Could you check a few things on this model? Use its own coordinates, in mm. Face numbers are marked on the shaded views. A direction names the side the tool comes from. Give positions to 0.01 mm unless a question says otherwise; leave off trailing zeros. Order: outer loops, then holes, each group sorted by start corner. A loop starts at its lowest first (then second) coordinate and runs counter-clockwise, first axis right, second up. Notation, with made-up numbers: (-14.5, 64) -> (-2.5, 64) arc R11 cw to (-2.5, 68) -> close; hole circle Ø6 at (47, 81). An arc over 180 degrees is marked (long way). One line per item, written item: value.
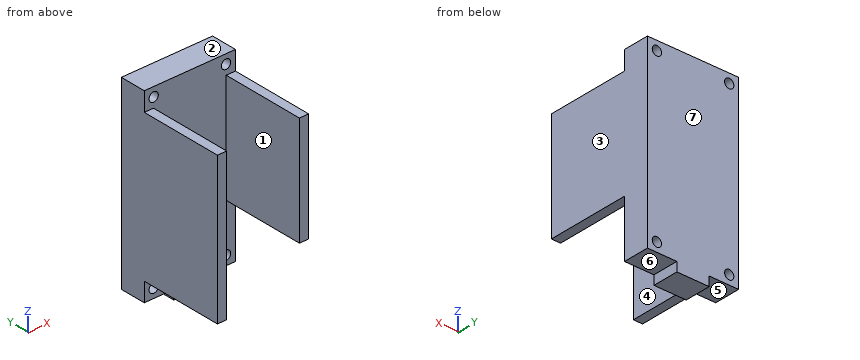
```python
from build123d import *

# Parameters (mm, degrees)
SKETCH1_W           = 25.0698
SKETCH1_H           = 51.054
SKETCH1_R           = 1.27
BOSS_EXTRUDE1_DEPTH = 7.1628
SKETCH2_W           = 2.54
SKETCH2_H           = 40.64
SKETCH2_H_2         = 30.1244
BOSS_EXTRUDE2_DEPTH = 22.86
SKETCH3_W           = 8.9
SKETCH3_H           = 7.1628
BOSS_EXTRUDE3_DEPTH = 2.54


with BuildPart() as part:
    # Sketch1 → Boss-Extrude1 (new body)
    with BuildSketch(Plane(origin=(0, 0, 0), x_dir=(1, 0, 0), z_dir=(0, 1, 0))):
        Rectangle(SKETCH1_W, SKETCH1_H)
        with Locations(Location((9.9441, 23.0124, 0), (0, 0, 270))):
            Circle(SKETCH1_R, mode=Mode.SUBTRACT)
        with Locations(Location((-9.9441, 23.0124, 0), (0, 0, 90))):
            Circle(SKETCH1_R, mode=Mode.SUBTRACT)
        with Locations(Location((9.9441, -23.0124, 0), (0, 0, 90))):
            Circle(SKETCH1_R, mode=Mode.SUBTRACT)
        with Locations(Location((-9.9441, -23.0124, 0), (0, 0, 270))):
            Circle(SKETCH1_R, mode=Mode.SUBTRACT)
    extrude(amount=BOSS_EXTRUDE1_DEPTH)

    # Sketch2 → Boss-Extrude2 (add)
    with BuildSketch(Plane.XZ):
        with Locations((-11.2649, 0)):
            Rectangle(SKETCH2_W, SKETCH2_H)
        with Locations((11.2649, 5.2578)):
            Rectangle(SKETCH2_W, SKETCH2_H_2)
    extrude(amount=BOSS_EXTRUDE2_DEPTH)

    # Sketch3 → Boss-Extrude3 (add)
    with BuildSketch(Plane(origin=(0, 0, -25.527), x_dir=(-1, 0, 0), z_dir=(0, 0, -1))):
        with Locations((0, 3.5814)):
            Rectangle(SKETCH3_W, SKETCH3_H)
    extrude(amount=BOSS_EXTRUDE3_DEPTH)


solid = part.part
```
1) If I drill on line 1 along X through (y, z) = (-6.5, 3.5); line 2 along Z through (x, y) = (-11, 5); line 3 along X through (y, z) = (-10.5, -16), over which ranges is the centre line in solid material (lowest first)?
Answer below:
line 1: x = -12.53 to -9.99, 9.99 to 12.53
line 2: z = -25.53 to -23.72, -22.31 to 22.31, 23.72 to 25.53
line 3: x = -12.53 to -9.99
2) We'd pull the mould along X, two halves only. Please class the marked faces 1, 2 and 3: +X half, -X half, draft (parallel to the pull), parting line (faces both ways), or undercut.
Answer below:
face 1: undercut
face 2: draft
face 3: +X half
3) Suppose I cut it at A-A, the plane y = -15. Write out the boundary of the cut face in (x, z), then the cut area to 3 significant figures.
Answer below:
outline: (-12.53, -20.32) -> (-9.99, -20.32) -> (-9.99, 20.32) -> (-12.53, 20.32) -> close; (9.99, -9.8) -> (12.53, -9.8) -> (12.53, 20.32) -> (9.99, 20.32) -> close
area: 180 mm2
4) Suppose I cut it at D-D, the plane y = 1. Write out the boundary of the cut face in (x, z).
Answer below:
outline: (-12.53, -25.53) -> (-4.45, -25.53) -> (-4.45, -28.07) -> (4.45, -28.07) -> (4.45, -25.53) -> (12.53, -25.53) -> (12.53, 25.53) -> (-12.53, 25.53) -> close; hole circle Ø2.54 at (-9.94, -23.01); hole circle Ø2.54 at (-9.94, 23.01); hole circle Ø2.54 at (9.94, -23.01); hole circle Ø2.54 at (9.94, 23.01)
5) Suppose I cut it at B-B, the plane z = 8.5. Write out the boundary of the cut face in (x, y).
Answer below:
outline: (-12.53, -22.86) -> (-9.99, -22.86) -> (-9.99, 0) -> (9.99, 0) -> (9.99, -22.86) -> (12.53, -22.86) -> (12.53, 7.16) -> (-12.53, 7.16) -> close
6) Suppose I cut it at C-C, the plane x = -3.25. Write out the boundary of the cut face in (y, z), then the cut area to 3 significant figures.
Answer below:
outline: (0, -28.07) -> (7.16, -28.07) -> (7.16, 25.53) -> (0, 25.53) -> close
area: 384 mm2
7) For P1, Ø3, axis at y = 4.5, z = -26.5, coming from the -X side; P2, Ø3.5, axis at x = 7, y = 3.5, coming from the -Z side; P3, Ø3, axis at x = 9.94, z = 23.01, coming from the -Y side; P4, Ø1.3, axis at x = -11.5, y = -17, coming from the -Z side, each with a flat end and sliding along its axis, tell me the tip position at first contact or that it passes through.
Answer below:
P1: stops at x = -12.53
P2: stops at z = -25.53
P3: stops at y = 0
P4: stops at z = -20.32
8) For the marked faces 4, 5, 6 and 7, which set-ups out of +Z, -Z, +X, -X, +Y, -Y let a thin tool reach every point of the face, with its end or its side?
Answer below:
face 4: +Z, -Z, -Y
face 5: -Z, -X, +Y, -Y
face 6: -Z, +X, +Y, -Y
face 7: +Z, -Z, +X, -X, +Y
